Can you work these out from the model? Positions are in its coordinate system, mm. Round coordinates to 2 decimals unless told otherwise and drop trailing zeros. Write each loop counter-clockwise with the first axis right and the second up, starting at its lowest first coordinate (ties: lowest second). Pieces come first, ordered by that corner, then holes.
Q1. If we section it at C-C (x = 0): Please give me the cut outline in (y, z) (3 decimals).
Q2. If we section it at B-B (y = -6.6): Please give me the cut outline in (x, z) (3 decimals), plus the area to 3 significant figures.
Q3. If we section it at A-A (z = 2.15): Please give me the cut outline in (x, y) (3 decimals).
Q4. Please list where these lines run through material, in increasing order: line 1 along Y through (x, z) = (0, 1.8) (3 decimals); line 2 along X through (y, z) = (9.25, 2.3); line 3 along Y through (x, z) = (-0.75, 0.95).
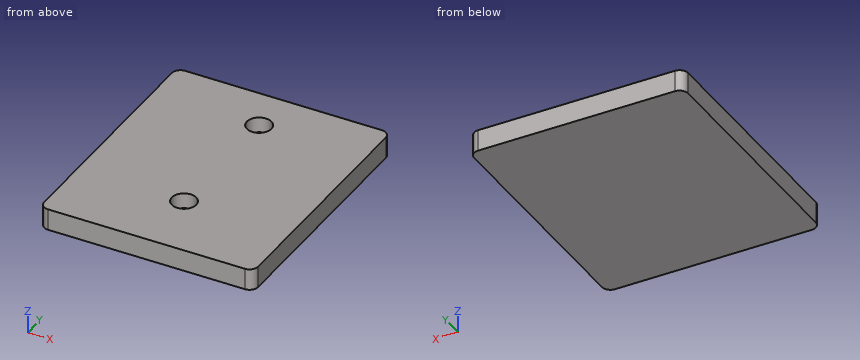
Autodesk Fusion 360 part; units mm, degrees
sketch "Sketch1" plane through (0, 0, 0) normal (0, 0, 1) x (1, 0, 0)
  line L0 (-12.45, 14.6) -> (12.45, 14.6)
  line L1 (12.45, 14.6) -> (12.45, -14.6)
  line L2 (12.45, -14.6) -> (-12.45, -14.6)
  line L3 (-12.45, -14.6) -> (-12.45, 14.6)
  line L4 (-12.45, -14.6) -> (12.45, 14.6) construction
  circle A0 centre (0, -6.6) radius 1.425
  circle A1 centre (0, -6.6) radius 2.75
  line L5 (0, 14.6) -> (0, -14.6) construction
  circle A2 centre (0, 9.4) radius 1.425
  circle A3 centre (0, 9.4) radius 2.75
  dimension "d1" = 24.9
  dimension "d2" = 29.2
  dimension "d92" = 2.85
  dimension "d98" = 5.5
  dimension "d141" = 8
  dimension "d142" = 16
extrude "Extrude1" add sketch "Sketch1" along normal blind 2.5 contours L0 L1 L2 L3 | A0 | A1 | A2 | A3
extrude "Extrude2" cut sketch "Sketch1" against normal blind 1.8 from surface at 2.5 contours A0 | A2
fillet "Fillet1" radius 1 4 edges at (-12.45, 14.6, 1.25) (12.45, 14.6, 1.25) (-12.45, -14.6, 1.25) (12.45, -14.6, 1.25)
A:
1. outline: (-14.6, 0) - (14.6, 0) - (14.6, 2.5) - (10.825, 2.5) - (10.825, 0.7) - (7.975, 0.7) - (7.975, 2.5) - (-5.175, 2.5) - (-5.175, 0.7) - (-8.025, 0.7) - (-8.025, 2.5) - (-14.6, 2.5) - close
2. outline: (-12.45, 0) - (12.45, 0) - (12.45, 2.5) - (1.425, 2.5) - (1.425, 0.7) - (-1.425, 0.7) - (-1.425, 2.5) - (-12.45, 2.5) - close
2. area: 57.1 mm2
3. outline: (-12.45, -13.6) arc R1 ccw to (-11.45, -14.6) - (11.45, -14.6) arc R1 ccw to (12.45, -13.6) - (12.45, 13.6) arc R1 ccw to (11.45, 14.6) - (-11.45, 14.6) arc R1 ccw to (-12.45, 13.6) - close; hole circle Ø2.85 at (0, -6.6); hole circle Ø2.85 at (0, 9.4)
4. line 1: y = -14.6 to -8.025, -5.175 to 7.975, 10.825 to 14.6
4. line 2: x = -12.45 to -1.42, 1.42 to 12.45
4. line 3: y = -14.6 to -7.81, -5.39 to 8.19, 10.61 to 14.6
